Could you check a few things on this model? Use its own coordinates, in mm. Give positions to 0.01 mm unless a question says otherwise; leave off trailing zeros. Order: outer loops, then holes, each group sorted by start corner. A loop starts at its lowest first (then second) coordinate and runs counter-clockwise, first axis right, second up. Notation, with made-up numbers: M 31,1.5 L 80,1.5 A6 cw 80,10.5 Z; hole C 79.25,47 d8. An arc over 180 degrees is marked long. Use a Markdown table: item, result. Add a question column.
```python
from build123d import *

# Parameters (mm, degrees)
SKETCH1_R               = 2.6035
BOSS_EXTRUDE1_DEPTH     = 304.8
SKETCH2_W               = 16.257599062
SKETCH2_H               = 27.586789262
CUT_EXTRUDE1_DEPTH      = 1.778
CUT_EXTRUDE1_DEPTH_BACK = 26.162


with BuildPart() as part:
    # Sketch1 → Boss-Extrude1 (new body, symmetric)
    with BuildSketch(Plane.XY):
        with BuildLine():
            Line((-7.179650497, -8.645192506), (-3.952270251, -5.423690499))
            ThreePointArc((-3.952270251, -5.423690499), (-2.922936451, -4.736929036), (-1.709253557, -4.4958))
            Line((-1.709253557, -4.4958), (1.709253557, -4.4958))
            ThreePointArc((1.709253557, -4.4958), (2.922936451, -4.736929036), (3.952270251, -5.423690499))
            Line((3.952270251, -5.423690499), (7.179650497, -8.645192506))
            ThreePointArc((7.179650497, -8.645192506), (7.41473083, -9.822813117), (6.416408329, -10.4902))
            Line((6.416408329, -10.4902), (4.287512407, -10.4902))
            ThreePointArc((4.287512407, -10.4902), (3.54574862, -10.79744862), (3.2385, -11.539212407))
            Line((3.2385, -11.539212407), (3.2385, -11.650987593))
            ThreePointArc((3.2385, -11.650987593), (3.54574862, -12.39275138), (4.287512407, -12.7))
            Line((4.287512407, -12.7), (5.317126718, -12.7))
            ThreePointArc((5.317126718, -12.7), (5.825126718, -12.192), (6.333126718, -12.7))
            Line((6.333126718, -12.7), (9.550443118, -12.7))
            ThreePointArc((9.550443118, -12.7), (10.058366869, -12.192000006), (10.566443095, -12.699847501))
            ThreePointArc((10.566443095, -12.699847501), (12.082537762, -12.08250727), (12.699846982, -10.566399977))
            ThreePointArc((12.699846982, -10.566399977), (12.192000006, -10.058323491), (12.7, -9.5504))
            Line((12.7, -9.5504), (12.7, -6.3330836))
            ThreePointArc((12.7, -6.3330836), (12.192, -5.8250836), (12.7, -5.3170836))
            Line((12.7, -5.3170836), (12.7, -4.287469289))
            ThreePointArc((12.7, -4.287469289), (12.39275138, -3.545705502), (11.650987593, -3.238456882))
            Line((11.650987593, -3.238456882), (11.539212407, -3.238456882))
            ThreePointArc((11.539212407, -3.238456882), (10.79744862, -3.545705502), (10.4902, -4.287469289))
            Line((10.4902, -4.287469289), (10.4902, -6.402089023))
            ThreePointArc((10.4902, -6.402089023), (9.856505071, -7.351067942), (8.737131347, -7.129408934))
            Line((8.737131347, -7.129408934), (5.441005833, -3.840816462))
            ThreePointArc((5.441005833, -3.840816462), (4.750877967, -2.809883091), (4.5085, -1.593185507))
            Line((4.5085, -1.593185507), (4.5085, 1.593185507))
            ThreePointArc((4.5085, 1.593185507), (4.750877967, 2.809883091), (5.441005833, 3.840816462))
            Line((5.441005833, 3.840816462), (8.737131347, 7.129408934))
            ThreePointArc((8.737131347, 7.129408934), (9.856505071, 7.351067942), (10.4902, 6.402089023))
            Line((10.4902, 6.402089023), (10.4902, 4.287469289))
            ThreePointArc((10.4902, 4.287469289), (10.79744862, 3.545705502), (11.539212407, 3.238456882))
            Line((11.539212407, 3.238456882), (11.650987593, 3.238456882))
            ThreePointArc((11.650987593, 3.238456882), (12.39275138, 3.545705502), (12.7, 4.287469289))
            Line((12.7, 4.287469289), (12.7, 5.3170836))
            ThreePointArc((12.7, 5.3170836), (12.192, 5.8250836), (12.7, 6.3330836))
            Line((12.7, 6.3330836), (12.7, 9.5504))
            ThreePointArc((12.7, 9.5504), (12.192000006, 10.058323491), (12.699846982, 10.566399977))
            ThreePointArc((12.699846982, 10.566399977), (12.082537762, 12.08250727), (10.566443095, 12.699847501))
            ThreePointArc((10.566443095, 12.699847501), (10.058366869, 12.192000006), (9.550443118, 12.7))
            Line((9.550443118, 12.7), (6.333126718, 12.7))
            ThreePointArc((6.333126718, 12.7), (5.825126718, 12.192), (5.317126718, 12.7))
            Line((5.317126718, 12.7), (4.287512407, 12.7))
            ThreePointArc((4.287512407, 12.7), (3.54574862, 12.39275138), (3.2385, 11.650987593))
            Line((3.2385, 11.650987593), (3.2385, 11.539212407))
            ThreePointArc((3.2385, 11.539212407), (3.54574862, 10.79744862), (4.287512407, 10.4902))
            Line((4.287512407, 10.4902), (6.476788598, 10.4902))
            ThreePointArc((6.476788598, 10.4902), (7.432222385, 9.85140422), (7.207036008, 8.724370562))
            Line((7.207036008, 8.724370562), (3.898272566, 5.423169045))
            ThreePointArc((3.898272566, 5.423169045), (2.869120213, 4.736787962), (1.655778399, 4.4958))
            Line((1.655778399, 4.4958), (-1.655778399, 4.4958))
            ThreePointArc((-1.655778399, 4.4958), (-2.869120213, 4.736787962), (-3.898272566, 5.423169045))
            Line((-3.898272566, 5.423169045), (-7.207036008, 8.724370562))
            ThreePointArc((-7.207036008, 8.724370562), (-7.432222385, 9.85140422), (-6.476788598, 10.4902))
            Line((-6.476788598, 10.4902), (-4.287512407, 10.4902))
            ThreePointArc((-4.287512407, 10.4902), (-3.54574862, 10.79744862), (-3.2385, 11.539212407))
            Line((-3.2385, 11.539212407), (-3.2385, 11.650987593))
            ThreePointArc((-3.2385, 11.650987593), (-3.54574862, 12.39275138), (-4.287512407, 12.7))
            Line((-4.287512407, 12.7), (-5.317126718, 12.7))
            ThreePointArc((-5.317126718, 12.7), (-5.825126718, 12.192), (-6.333126718, 12.7))
            Line((-6.333126718, 12.7), (-9.550443118, 12.7))
            ThreePointArc((-9.550443118, 12.7), (-10.058366869, 12.192000006), (-10.566443095, 12.699847501))
            ThreePointArc((-10.566443095, 12.699847501), (-12.082537762, 12.08250727), (-12.699846982, 10.566399977))
            ThreePointArc((-12.699846982, 10.566399977), (-12.192000006, 10.058323491), (-12.7, 9.5504))
            Line((-12.7, 9.5504), (-12.7, 6.3330836))
            ThreePointArc((-12.7, 6.3330836), (-12.192, 5.8250836), (-12.7, 5.3170836))
            Line((-12.7, 5.3170836), (-12.7, 4.287469289))
            ThreePointArc((-12.7, 4.287469289), (-12.39275138, 3.545705502), (-11.650987593, 3.238456882))
            Line((-11.650987593, 3.238456882), (-11.539212407, 3.238456882))
            ThreePointArc((-11.539212407, 3.238456882), (-10.79744862, 3.545705502), (-10.4902, 4.287469289))
            Line((-10.4902, 4.287469289), (-10.4902, 6.402089023))
            ThreePointArc((-10.4902, 6.402089023), (-9.856505071, 7.351067942), (-8.737131347, 7.129408934))
            Line((-8.737131347, 7.129408934), (-5.441005833, 3.840816462))
            ThreePointArc((-5.441005833, 3.840816462), (-4.750877967, 2.809883091), (-4.5085, 1.593185507))
            Line((-4.5085, 1.593185507), (-4.5085, -1.593185507))
            ThreePointArc((-4.5085, -1.593185507), (-4.750877967, -2.809883091), (-5.441005833, -3.840816462))
            Line((-5.441005833, -3.840816462), (-8.737131347, -7.129408934))
            ThreePointArc((-8.737131347, -7.129408934), (-9.856505071, -7.351067942), (-10.4902, -6.402089023))
            Line((-10.4902, -6.402089023), (-10.4902, -4.287469289))
            ThreePointArc((-10.4902, -4.287469289), (-10.79744862, -3.545705502), (-11.539212407, -3.238456882))
            Line((-11.539212407, -3.238456882), (-11.650987593, -3.238456882))
            ThreePointArc((-11.650987593, -3.238456882), (-12.39275138, -3.545705502), (-12.7, -4.287469289))
            Line((-12.7, -4.287469289), (-12.7, -5.3170836))
            ThreePointArc((-12.7, -5.3170836), (-12.192, -5.8250836), (-12.7, -6.3330836))
            Line((-12.7, -6.3330836), (-12.7, -9.5504))
            ThreePointArc((-12.7, -9.5504), (-12.192000006, -10.058323491), (-12.699846982, -10.566399977))
            ThreePointArc((-12.699846982, -10.566399977), (-12.082537762, -12.08250727), (-10.566443095, -12.699847501))
            ThreePointArc((-10.566443095, -12.699847501), (-10.058366869, -12.192000006), (-9.550443118, -12.7))
            Line((-9.550443118, -12.7), (-6.333126718, -12.7))
            ThreePointArc((-6.333126718, -12.7), (-5.825126718, -12.192), (-5.317126718, -12.7))
            Line((-5.317126718, -12.7), (-4.287512407, -12.7))
            ThreePointArc((-4.287512407, -12.7), (-3.54574862, -12.39275138), (-3.2385, -11.650987593))
            Line((-3.2385, -11.650987593), (-3.2385, -11.539212407))
            ThreePointArc((-3.2385, -11.539212407), (-3.54574862, -10.79744862), (-4.287512407, -10.4902))
            Line((-4.287512407, -10.4902), (-6.416408329, -10.4902))
            ThreePointArc((-6.416408329, -10.4902), (-7.41473083, -9.822813117), (-7.179650497, -8.645192506))
        make_face()
        Circle(SKETCH1_R, mode=Mode.SUBTRACT)
    extrude(amount=BOSS_EXTRUDE1_DEPTH, both=True)

    # Sketch2 → Cut-Extrude1 (cut, two sides)
    with BuildSketch(Plane(origin=(12.7, 0, 0), x_dir=(0, 0, -1), z_dir=(1, 0, 0))) as cut_extrude1_sk:
        Polygon((-56.586481007, -14.234528627), (310.743066166, -14.234528627), (310.743066166, 13.643777343), (-56.586481007, 13.643777343), (-101.042247833, 13.643777343), (-101.042247833, -14.234528627), align=None)
        with Locations((-297.347005301, -0.441133996)):
            Rectangle(SKETCH2_W, SKETCH2_H)
    extrude(amount=CUT_EXTRUDE1_DEPTH, mode=Mode.SUBTRACT)
    extrude(cut_extrude1_sk.sketch, amount=-CUT_EXTRUDE1_DEPTH_BACK, mode=Mode.SUBTRACT)


solid = part.part
```
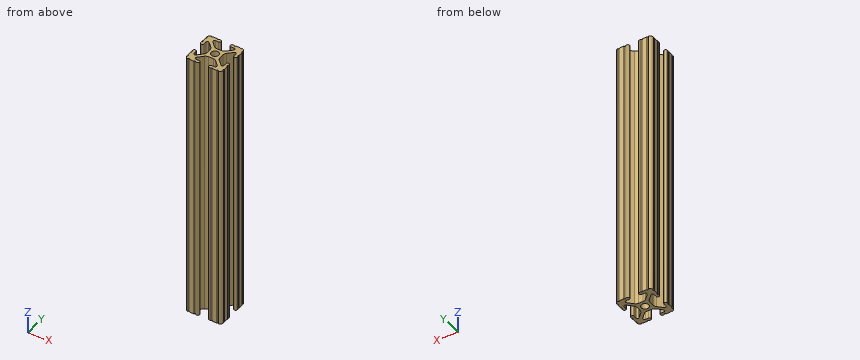
1) Suppose I cut it at B-B on y = 0. Please give me the cut outline in (x, z), and give its area (3 significant figures).
2) Suppose I cut it at A-A on x = 0. Please give me the cut outline in (y, z).
3) For pin 1 (2.5 mm diameter, centred on y = 0, z = 241.5, fed in from -X); pin 2 (1.1 mm diameter, centred on x = 5.5, z = 173.5, fed in from +Y); pin 3 (1.7 mm diameter, centred on x = -0.5, z = 222.5, fed in from +Y); pin 4 (1 mm diameter, centred on y = 0.5, z = 236.5, fed in from +X), each with a flat end and sliding along its axis, tell me the tip position at first contact or that it passes through.
4) Please list where these lines run through material, in increasing order: line 1 (Y direction, x = 0, z = 199); line 2 (X direction, y = 0, z = 250.5); line 3 (X direction, y = -9.25, z = 221.5). Write a range as from..to.
Values found:
| question | item | result |
|---|---|---|
| 1 | outline | M -4.51,101.04 L -2.6,101.04 L -2.6,289.22 L -4.51,289.22 Z; M 2.6,101.04 L 4.51,101.04 L 4.51,289.22 L 2.6,289.22 Z |
| 1 | area | 717 mm^2 |
| 2 | outline | M -4.5,101.04 L -2.6,101.04 L -2.6,289.22 L -4.5,289.22 Z; M 2.6,101.04 L 4.5,101.04 L 4.5,289.22 L 2.6,289.22 Z |
| 3 | pin 1 | stops at x = -4.51 |
| 3 | pin 2 | stops at y = 12.7 |
| 3 | pin 3 | stops at y = 4.5 |
| 3 | pin 4 | stops at x = 4.51 |
| 4 | line 1 | y = -4.5..-2.6, 2.6..4.5 |
| 4 | line 2 | x = -4.51..-2.6, 2.6..4.51 |
| 4 | line 3 | x = -12.7..-7.48, 7.48..12.7 |
